The listing builds one solid part. Answer for the finished solid, in the listing's coordinates (mm). Face numbers are marked on the shaded views. A direction names the side the tool comes from. Coordinates: 2 decimals unless noted, no trailing zeros. Order: outer loops, then holes, each group sorted by start corner. A loop starts at its lowest first (then second) coordinate and runs counter-clockwise, first axis right, second up. Notation, with made-up numbers: (40, 38.5) -> (61, 38.5) arc R24 ccw to (61, 68.5) -> close; hole circle Ø8 at (52, -24.75). An arc over 180 degrees is marked (long way). Return JSON: item names as keys, results as strings.
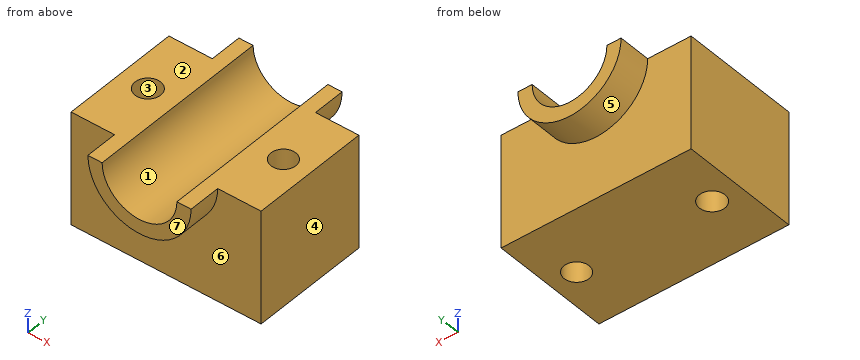
```python
from build123d import *

# Parameters (mm, degrees)
F1_DEPTH = 23.368
F2_DEPTH = 36.068
F3_R     = 5.00372
F3_R_2   = 4.870923
F4_DEPTH = 64.008


with BuildPart() as f1:
    # F0 (on Front) → F1 (new body, symmetric)
    with BuildSketch(Plane.XZ):
        with BuildLine():
            Line((-37.199613, -22.161454), (37.199613, -22.161454))
            Line((37.199613, -22.161454), (37.199613, 22.161454))
            Line((37.199613, 22.161454), (20.20446, 22.161454))
            ThreePointArc((20.20446, 22.161454), (0, 1.956994), (-20.20446, 22.161454))
            Line((-20.20446, 22.161454), (-37.199613, 22.161454))
            Line((-37.199613, 22.161454), (-37.199613, -22.161454))
        make_face()
    extrude(amount=F1_DEPTH, both=True)

    # F0 (on Front) → F2 (join, symmetric)
    with BuildSketch(Plane.XZ):
        with BuildLine():
            ThreePointArc((-20.20446, 22.161454), (0, 1.956994), (20.20446, 22.161454))
            Line((20.20446, 22.161454), (14.641577, 22.161454))
            ThreePointArc((14.641577, 22.161454), (0, 7.519877), (-14.641577, 22.161454))
            Line((-14.641577, 22.161454), (-20.20446, 22.161454))
        make_face()
    extrude(amount=F2_DEPTH, both=True)

    # F3 (on face) → F4 (cut)
    with BuildSketch(Plane.XY.offset(22.161454)):
        with Locations((-26.294084, 0)):
            Circle(F3_R)
        with Locations((26.79375, 0)):
            Circle(F3_R_2)
    extrude(amount=-F4_DEPTH, mode=Mode.SUBTRACT)


solid = f1.part
```
Item 1: Which of the six approach directions +Z, -Z, +X, -X, +Y, -Y give full straight-line access (tool end or side, diameter ignored) to the marked faces 5, 6 and 7?
Answer list:
{"face 5": "-Z, +Y", "face 6": "-Z, -Y", "face 7": "+Z, -Z, +X, -X, -Y"}
Item 2: Find the intervals of material crossed by probe 1 along Y at (x, z) = (-26.5, 6); probe 2 along Y at (x, z) = (-28, -2); probe 3 along Y at (x, z) = (-4, -16), in increasing order.
Answer list:
{"probe 1": "-23.37 to -5, 5 to 23.37", "probe 2": "-23.37 to -4.7, 4.7 to 23.37", "probe 3": "-23.37 to 23.37"}
Item 3: Determine the mould class of the marked faces 1, 2, 3 and 4 for opening direction X: pulls with the +X half, pulls with the -X half, needs draft (parallel to the pull), parting line crosses it, or undercut.
Answer list:
{"face 1": "undercut", "face 2": "needs draft", "face 3": "undercut", "face 4": "pulls with the +X half"}
Item 4: The part is cut by section C-C on x = 0. Determine the outline of the cut face in (y, z).
Answer list:
{"outline": "(-36.07, 1.96) -> (-23.37, 1.96) -> (-23.37, -22.16) -> (23.37, -22.16) -> (23.37, 1.96) -> (36.07, 1.96) -> (36.07, 7.52) -> (-36.07, 7.52) -> close"}
Item 5: Flat-ended cylindrical pins translate along their axes: pin 1 (2 mm diameter, centred on x = -20.5, z = -6.5, fed in from -Y); pin 2 (6 mm diameter, centred on x = 1.5, y = -24.5, fed in from +Z). Find the tip coordinate at first contact, or state that the pin passes through.
Answer list:
{"pin 1": "y = -23.37", "pin 2": "z = 8.23"}
Item 6: The part is cut by section D-D on z = -18. Determine the outline of the cut face in (x, y).
Answer list:
{"outline": "(-37.2, -23.37) -> (37.2, -23.37) -> (37.2, 23.37) -> (-37.2, 23.37) -> close; hole circle Ø10.01 at (-26.29, 0); hole circle Ø9.74 at (26.79, 0)"}
Item 7: The part is cut by section A-A on y = 0. Determine the outline of the cut face in (x, z).
Answer list:
{"outline": "(-37.2, -22.16) -> (-31.3, -22.16) -> (-31.3, 22.16) -> (-37.2, 22.16) -> close; (-21.29, -22.16) -> (21.92, -22.16) -> (21.92, 22.16) -> (14.64, 22.16) arc R14.64 cw to (-14.64, 22.16) -> (-21.29, 22.16) -> close; (31.66, -22.16) -> (37.2, -22.16) -> (37.2, 22.16) -> (31.66, 22.16) -> close"}
Item 8: The part is cut by section B-B on z = 16. Determine the outline of the cut face in (x, y).
Answer list:
{"outline": "(-37.2, -23.37) -> (-19.24, -23.37) -> (-19.24, -36.07) -> (-13.28, -36.07) -> (-13.28, 36.07) -> (-19.24, 36.07) -> (-19.24, 23.37) -> (-37.2, 23.37) -> close; (13.28, -36.07) -> (19.24, -36.07) -> (19.24, -23.37) -> (37.2, -23.37) -> (37.2, 23.37) -> (19.24, 23.37) -> (19.24, 36.07) -> (13.28, 36.07) -> close; hole circle Ø10.01 at (-26.29, 0); hole circle Ø9.74 at (26.79, 0)"}
